Geometry check sheet. Reference: the model listing, model coordinates, mm. Face numbers are marked on the shaded views. A direction names the side the tool comes from. Round coordinates to 2 decimals unless told otherwise and drop trailing zeros. Order: outer loops, then holes, each group sorted by start corner. A loop starts at its lowest first (then second) coordinate and runs counter-clockwise, first axis right, second up. Notation, with made-up numbers: (-32.5, 50.25) - (7.5, 50.25) arc R14 ccw to (7.5, 74.25) - close; hole circle Ø11 at (67.25, -9). An arc over 180 degrees is marked (long way). Return JSON: item names as keys, results as strings. Group by question number.
Q1. Tool access check on the marked faces 4, 5 and 6. Record the directions out of +Z, -Z, +X, -X, +Y, -Y that give a thin tool (end or side, any length) a straight path to the whole face; none if there is none.
Q2. Sectioned sample at B-B, the plane y = 0. Record the cut outline in (x, z), then the cut area to 3 significant figures.
Q3. Gauge pin test, flat ends, axial feed: pin 1 Ø3 at (x, z) = (11, -15) entering from +Y; pin 2 Ø1.2 at (y, z) = (8, -3) entering from -X; pin 3 Ø6 at (x, z) = (-9, -8.5) entering from +Y. Record the tip position at first contact, or that the pin passes through.
Q4. Draft check along Z on the marked faces 1, 2 and 3. Enter one of: pulls with the +Z half, pulls with the -Z half, needs draft (parallel to the pull), parting line crosses it, or undercut.
Q5. Material ranges on line 1 along Z through (x, y) = (-25, 0.5); line 2 along X through (y, z) = (-19.5, -8); line 3 along X through (y, z) = (0, -5.75), recorded low to high.
```python
from build123d import *

# Parameters (mm, degrees)
CUT_EXTRUDE1_START      = -0.7874
CUT_EXTRUDE1_DEPTH      = 14.3002
CIRPATTERN1_COUNT       = 16
SKETCH4_R               = 3.175
CUT_EXTRUDE2_DEPTH      = 43.478219515
CUT_EXTRUDE3_START      = 1.5875
SKETCH5_R               = 30.004447146
CUT_EXTRUDE3_DEPTH      = 20.32
CUT_EXTRUDE4_DEPTH      = 20.32
CUT_EXTRUDE4_DEPTH_BACK = 20.32
SKETCH6_W               = 6.35
SKETCH6_H               = 6.35


with BuildPart() as part:
    # Sketch2 → Revolve1 (revolve)
    with BuildSketch(Plane(origin=(0, 0, 0), x_dir=(0, 0, -1), z_dir=(1, 0, 0)), mode=Mode.PRIVATE) as revolve1_sk:
        with BuildLine():
            Line((-17.4625, 6.35), (17.4625, 6.35))
            Line((17.4625, 6.35), (17.4625, 27.3812))
            Line((17.4625, 27.3812), (16.27505, 27.3812))
            ThreePointArc((16.27505, 27.3812), (15.408504076, 26.591481572), (15.0876, 25.463839073))
            Line((15.0876, 25.463839073), (15.0876, 23.546478146))
            Line((15.0876, 23.546478146), (0.7874, 23.546478146))
            Line((0.7874, 23.546478146), (0.7874, 25.463839073))
            ThreePointArc((0.7874, 25.463839073), (0.466495924, 26.591481572), (-0.40005, 27.3812))
            Line((-0.40005, 27.3812), (-1.5875, 27.3812))
            Line((-1.5875, 27.3812), (-1.5875, 18.2626))
            Line((-1.5875, 18.2626), (-17.4625, 18.2626))
            Line((-17.4625, 18.2626), (-17.4625, 6.35))
        make_face()
    revolve(revolve1_sk.sketch.rotate(Axis((0, 0, 17.4625), (0, 0, -1)), 90), axis=Axis((0, 0, 17.4625), (0, 0, -1)))

    # Sketch3 → Cut-Extrude1 (cut)
    with BuildSketch(Plane.XY.offset(CUT_EXTRUDE1_START)):
        with BuildLine():
            Line((-1.630736704, 21.5265), (1.630736704, 21.5265))
            Line((1.630736704, 21.5265), (2.3241, 23.4315))
            ThreePointArc((2.3241, 23.4315), (0, 23.546478146), (-2.3241, 23.4315))
            Line((-2.3241, 23.4315), (-1.630736704, 21.5265))
        make_face()
    cut_extrude1 = extrude(amount=-CUT_EXTRUDE1_DEPTH, mode=Mode.SUBTRACT)

    # CirPattern1: Cut-Extrude1 ×16 about axis
    cirpattern1_axis = Axis((0, 0, 0), (0, 0, 1))
    for i in range(1, CIRPATTERN1_COUNT):
        add(cut_extrude1.rotate(cirpattern1_axis, i * 360 / CIRPATTERN1_COUNT), mode=Mode.SUBTRACT)

    # Sketch4 → Cut-Extrude2 (cut, through all)
    with BuildSketch(Plane(origin=(0, 0, 0), x_dir=(0, -1, 0), z_dir=(1, 0, 0))):
        with Locations(Location((0, -9.525, 0), (0, 0, 270))):
            Circle(SKETCH4_R)
    extrude(amount=CUT_EXTRUDE2_DEPTH, mode=Mode.SUBTRACT)

    # Sketch5 → Cut-Extrude3 (cut)
    with BuildSketch(Plane.XY.offset(CUT_EXTRUDE3_START)):
        Circle(SKETCH5_R)
    extrude(amount=CUT_EXTRUDE3_DEPTH, mode=Mode.SUBTRACT)

    # Sketch6 → Cut-Extrude4 (cut, two sides: drawn at the far end of the back side and taken through both)
    with BuildSketch(Plane.XY.offset(-CUT_EXTRUDE4_DEPTH_BACK)):
        with Locations((0, 6.35)):
            Rectangle(SKETCH6_W, SKETCH6_H)
    extrude(amount=CUT_EXTRUDE4_DEPTH + CUT_EXTRUDE4_DEPTH_BACK, mode=Mode.SUBTRACT)


solid = part.part
```
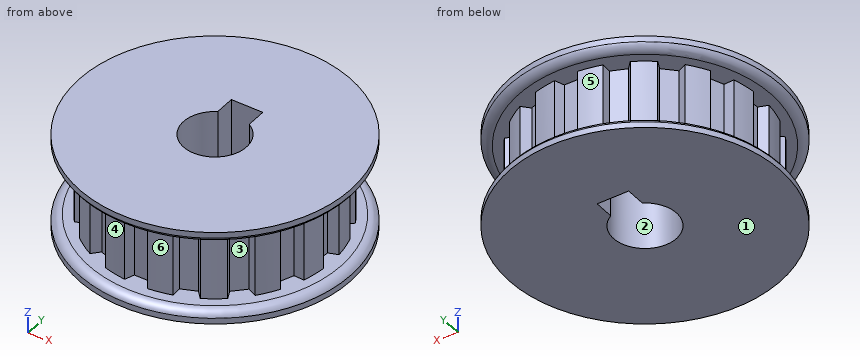
Reply:
{
 "1": {"face 4": "-X, -Y", "face 5": "-X, +Y", "face 6": "+X, -Y"},
 "2": {"outline": "(-27.38, -17.46) - (-6.35, -17.46) - (-6.35, 1.59) - (-27.38, 1.59) - (-27.38, 0.4) arc R2.14 ccw to (-25.46, -0.79) - (-21.53, -0.79) - (-21.53, -15.09) - (-25.46, -15.09) arc R2.14 ccw to (-27.38, -16.28) - close; (6.35, -17.46) - (27.38, -17.46) - (27.38, -16.28) arc R2.14 ccw to (25.46, -15.09) - (21.53, -15.09) - (21.53, -0.79) - (25.46, -0.79) arc R2.14 ccw to (27.38, 0.4) - (27.38, 1.59) - (6.35, 1.59) - close", "area": "631 mm^2"},
 "3": {"pin 1": "y = 25.41", "pin 2": "x = -20.23", "pin 3": "y = 22.77"},
 "4": {"face 1": "pulls with the -Z half", "face 2": "needs draft", "face 3": "undercut"},
 "5": {"line 1": "-17.46 to -15.09, -0.79 to 1.59", "line 2": "-13.2 to -9.96, -9.17 to 9.17, 9.96 to 13.2", "line 3": "-21.53 to -6.35, 6.35 to 21.53"}
}
